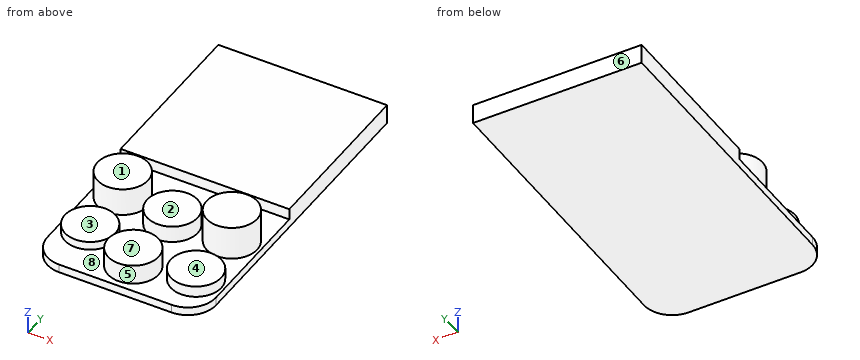
from build123d import *

# Parameters (mm, degrees)
F0_W     = 30
F0_H     = 30
F0_R     = 4.5
F1_DEPTH = 1.5
F2_DEPTH = 2
F3_DEPTH = 5
F4_DEPTH = 3
F5_DEPTH = 6
F6_DEPTH = 2
F7_DEPTH = 3.5
F8_DEPTH = 1.5


with BuildPart() as f1:
    # F0 (on Top) → F1 (new body)
    with BuildSketch(Plane.XY):
        with Locations((0, 3.183698)):
            Rectangle(F0_W, F0_H)
        with BuildLine():
            Line((15, -11.816302), (-15, -11.816302))
            Line((-15, -11.816302), (-15, -34.316302))
            ThreePointArc((-15, -34.316302), (-13.535534, -37.851836), (-10, -39.316302))
            Line((-10, -39.316302), (10, -39.316302))
            ThreePointArc((10, -39.316302), (13.535534, -37.851836), (15, -34.316302))
            Line((15, -34.316302), (15, -11.816302))
        make_face()
        with Locations((-10, -29.816302)):
            Circle(F0_R, mode=Mode.SUBTRACT)
        with Locations((-10, -19.816302)):
            Circle(F0_R, mode=Mode.SUBTRACT)
        with Locations((0, -33.816302)):
            Circle(F0_R, mode=Mode.SUBTRACT)
        with Locations((10, -31.816302)):
            Circle(F0_R, mode=Mode.SUBTRACT)
        with Locations((0, -21.816302)):
            Circle(F0_R, mode=Mode.SUBTRACT)
        with Locations((10, -20.816302)):
            Circle(F0_R, mode=Mode.SUBTRACT)
        with Locations((-10, -19.816302)):
            Circle(F0_R)
        with Locations((0, -21.816302)):
            Circle(F0_R)
        with Locations((10, -20.816302)):
            Circle(F0_R)
        with Locations((10, -31.816302)):
            Circle(F0_R)
        with Locations((0, -33.816302)):
            Circle(F0_R)
        with Locations((-10, -29.816302)):
            Circle(F0_R)
    extrude(amount=-F1_DEPTH)

    # F0 (on Top) → F2 (join)
    with BuildSketch(Plane.XY):
        with Locations((0, 3.183698)):
            Rectangle(F0_W, F0_H)
    extrude(amount=F2_DEPTH)

    # F0 (on Top) → F3 (join)
    with BuildSketch(Plane.XY):
        with Locations((-10, -19.816302)):
            Circle(F0_R)
    extrude(amount=F3_DEPTH)

    # F0 (on Top) → F4 (join)
    with BuildSketch(Plane.XY):
        with Locations((0, -21.816302)):
            Circle(F0_R)
    extrude(amount=F4_DEPTH)

    # F0 (on Top) → F5 (join)
    with BuildSketch(Plane.XY):
        with Locations((10, -20.816302)):
            Circle(F0_R)
    extrude(amount=F5_DEPTH)

    # F0 (on Top) → F6 (join)
    with BuildSketch(Plane.XY):
        with Locations((10, -31.816302)):
            Circle(F0_R)
    extrude(amount=F6_DEPTH)

    # F0 (on Top) → F7 (join)
    with BuildSketch(Plane.XY):
        with Locations((0, -33.816302)):
            Circle(F0_R)
    extrude(amount=F7_DEPTH)

    # F0 (on Top) → F8 (join)
    with BuildSketch(Plane.XY):
        with Locations((-10, -29.816302)):
            Circle(F0_R)
    extrude(amount=F8_DEPTH)


solid = f1.part
Model file for the job. Use its own axes, mm. Face numbers are marked on the shaded views. A direction names the side the tool comes from. Coordinates: 2 decimals unless noted, no trailing zeros. Order: outer loops, then holes, each group sorted by start corner. A loop starts at its lowest first (then second) coordinate and runs counter-clockwise, first axis right, second up. Notation, with made-up numbers: M 46,-34.5 L 52,-34.5 A17 ccw 52,-17.5 Z; hole C 30,-21.5 d11. An arc over 180 degrees is marked long. Return JSON: item names as keys, results as strings.
1. Tool access for the marked faces 1, 2, 3, 4 and 5: list every direction of +Z, -Z, +X, -X, +Y, -Y with a clear straight run to the whole face (end or side of a thin tool).
Ans:
{"face 1": "+Z, -X, +Y, -Y", "face 2": "+Z, +Y", "face 3": "+Z, -X, -Y", "face 4": "+Z, +X, -Y", "face 5": "+Z"}
2. Pull direction Y, two halves, no side cores. Call the marked faces 6, 7 and 8: +Y half, -Y half, draft (parallel to the pull), parting line (faces both ways), or undercut.
Ans:
{"face 6": "+Y half", "face 7": "draft", "face 8": "undercut"}
3. Saw through at B-B (y = -35). Give the cut face in (x, z), and give its area (3 significant figures).
Ans:
{"outline": "M -14.95,-1.5 L 14.95,-1.5 L 14.95,0 L 13.18,0 L 13.18,2 L 6.82,2 L 6.82,0 L 4.34,0 L 4.34,3.5 L -4.34,3.5 L -4.34,0 L -14.95,0 Z", "area": "88.0 mm^2"}
4. Saw through at A-A (x = 0). Give the cut face in (y, z), and give its area (3 significant figures).
Ans:
{"outline": "M -39.32,-1.5 L 18.18,-1.5 L 18.18,2 L -11.82,2 L -11.82,0 L -17.32,0 L -17.32,3 L -26.32,3 L -26.32,0 L -29.32,0 L -29.32,3.5 L -38.32,3.5 L -38.32,0 L -39.32,0 Z", "area": "205 mm^2"}
5. Drill centre lines: probe 1 along Y at (x, z) = (0, 1.5); probe 2 along Y at (x, z) = (3, 1.75); probe 3 along X at (y, z) = (-31.5, 0.25). Where is each one in solid material? Low to high.
Ans:
{"probe 1": "-38.32 to -29.32, -26.32 to -17.32, -11.82 to 18.18", "probe 2": "-37.17 to -30.46, -25.17 to -18.46, -11.82 to 18.18", "probe 3": "-14.17 to -5.83, -3.86 to 3.86, 5.51 to 14.49"}
6. Saw through at D-D (x = 11). Give the cut face in (y, z), and give its area (3 significant figures).
Ans:
{"outline": "M -39.22,-1.5 L 18.18,-1.5 L 18.18,2 L -11.82,2 L -11.82,0 L -16.43,0 L -16.43,6 L -25.2,6 L -25.2,0 L -27.43,0 L -27.43,2 L -36.2,2 L -36.2,0 L -39.22,0 Z", "area": "216 mm^2"}
7. Flat gauge pins, fed straight in: pin 1 (1.6 mm diameter, centred on x = -1.5, z = 1.5, fed in from -Y); pin 2 (2.5 mm diameter, centred on x = -9, y = -28, fed in from +Z); pin 3 (1 mm diameter, centred on x = -6.5, y = -13.5, fed in from +Z); pin 4 (1.5 mm diameter, centred on x = 2.5, z = 2.5, fed in from +Y). Where does each tip first touch, or does it go through?
Ans:
{"pin 1": "y = -38.26", "pin 2": "z = 1.5", "pin 3": "z = 0", "pin 4": "y = 18.18"}
8. Saw through at C-C (y = -9.5). Give the cut face in (x, z).
Ans:
{"outline": "M -15,-1.5 L 15,-1.5 L 15,2 L -15,2 Z"}
